Source: CAD feature listing. Evaluate the final solid. Frame: model axes, mm. A direction names the side the tool comes from. Give positions to 0.01 mm unless a question says otherwise; leave off trailing zeros. Order: outer loops, then holes, each group sorted by start corner. A loop starts at its lowest first (then second) coordinate and runs counter-clockwise, first axis right, second up.
from build123d import *

# Parameters (mm, degrees)
SKETCH1_R           = 10
SKETCH1_R_2         = 5.5
BOSS_EXTRUDE1_DEPTH = 2
SKETCH3_R           = 3
BOSS_EXTRUDE2_DEPTH = 12
SKETCH4_R           = 10
SKETCH4_R_2         = 3
BOSS_EXTRUDE3_DEPTH = 2
CHAMFER2_SIZE       = 1
CHAMFER4_SIZE       = 0.5
CUT_EXTRUDE1_REACH  = 6
SKETCH5_R           = 0.75
SKETCH6_R           = 6.25
SKETCH6_R_2         = 5.5
BOSS_EXTRUDE4_DEPTH = 26
CUT_EXTRUDE2_REACH  = 32
SKETCH7_R           = 0.75
SKETCH9_R           = 17.358770913
CUT_EXTRUDE3_DEPTH  = 28


with BuildPart() as part:
    # Sketch1 → Boss-Extrude1 (new body)
    with BuildSketch(Plane.XY):
        Circle(SKETCH1_R)
        Circle(SKETCH1_R_2, mode=Mode.SUBTRACT)
    extrude(amount=BOSS_EXTRUDE1_DEPTH)



with BuildPart() as body_2:
    # Sketch3 → Boss-Extrude2 (new body)
    with BuildSketch(Plane(origin=(0, 0, 0), x_dir=(-1, 0, 0), z_dir=(0, 0, -1))):
        Circle(SKETCH3_R)
    extrude(amount=BOSS_EXTRUDE2_DEPTH)


with BuildPart() as part_1:
    add(part.part)

    add(body_2.part)  # Boss-Extrude3 merges body 2
    # Sketch4 → Boss-Extrude3 (add)
    with BuildSketch(Plane(origin=(0, 0, 0), x_dir=(-1, 0, 0), z_dir=(0, 0, -1))):
        Circle(SKETCH4_R)
        Circle(SKETCH4_R_2, mode=Mode.SUBTRACT)
    extrude(amount=BOSS_EXTRUDE3_DEPTH)

    # Chamfer2
    chamfer2_edges = [part_1.edges().sort_by_distance(p)[0] for p in [
        (3, 0, -2),
    ]]
    chamfer(chamfer2_edges, length=CHAMFER2_SIZE)

    # Chamfer4
    chamfer4_edges = [part_1.edges().sort_by_distance(p)[0] for p in [
        (3, 0, -12),
    ]]
    chamfer(chamfer4_edges, length=CHAMFER4_SIZE)

    # Sketch5 → Cut-Extrude1 (cut, up to next)
    with BuildSketch(Plane(origin=(0, 0, -2), x_dir=(-1, 0, 0), z_dir=(0, 0, -1)), mode=Mode.PRIVATE) as cut_extrude1_sk1:
        with Locations((-8.5, 0)):
            Circle(SKETCH5_R)
    cut_extrude1_tool1 = extrude(cut_extrude1_sk1.sketch, amount=-CUT_EXTRUDE1_REACH, mode=Mode.PRIVATE) & part_1.part
    add(cut_extrude1_tool1.solids().sort_by_distance((8.5, 0, -2))[0], mode=Mode.SUBTRACT)
    # Sketch5 → Cut-Extrude1 (cut, up to next)
    with BuildSketch(Plane(origin=(0, 0, -2), x_dir=(-1, 0, 0), z_dir=(0, 0, -1)), mode=Mode.PRIVATE) as cut_extrude1_sk2:
        with Locations((8.5, 0)):
            Circle(SKETCH5_R)
    cut_extrude1_tool2 = extrude(cut_extrude1_sk2.sketch, amount=-CUT_EXTRUDE1_REACH, mode=Mode.PRIVATE) & part_1.part
    add(cut_extrude1_tool2.solids().sort_by_distance((-8.5, 0, -2))[0], mode=Mode.SUBTRACT)

    # Sketch6 → Boss-Extrude4 (add)
    with BuildSketch(Plane.XY.offset(2)):
        Circle(SKETCH6_R)
        Circle(SKETCH6_R_2, mode=Mode.SUBTRACT)
    extrude(amount=BOSS_EXTRUDE4_DEPTH)

    # Sketch7 → Cut-Extrude2 (cut, up to next)
    with BuildSketch(Plane(origin=(0, 0, -2), x_dir=(-1, 0, 0), z_dir=(0, 0, -1)), mode=Mode.PRIVATE) as cut_extrude2_sk1:
        with Locations((0, 7.5)):
            Circle(SKETCH7_R)
    cut_extrude2_tool1 = extrude(cut_extrude2_sk1.sketch, amount=-CUT_EXTRUDE2_REACH, mode=Mode.PRIVATE) & part_1.part
    add(cut_extrude2_tool1.solids().sort_by_distance((0, 7.5, -2))[0], mode=Mode.SUBTRACT)
    # Sketch7 → Cut-Extrude2 (cut, up to next)
    with BuildSketch(Plane(origin=(0, 0, -2), x_dir=(-1, 0, 0), z_dir=(0, 0, -1)), mode=Mode.PRIVATE) as cut_extrude2_sk2:
        with Locations((6.495190528, -3.75)):
            Circle(SKETCH7_R)
    cut_extrude2_tool2 = extrude(cut_extrude2_sk2.sketch, amount=-CUT_EXTRUDE2_REACH, mode=Mode.PRIVATE) & part_1.part
    add(cut_extrude2_tool2.solids().sort_by_distance((-6.495191, -3.75, -2))[0], mode=Mode.SUBTRACT)
    # Sketch7 → Cut-Extrude2 (cut, up to next)
    with BuildSketch(Plane(origin=(0, 0, -2), x_dir=(-1, 0, 0), z_dir=(0, 0, -1)), mode=Mode.PRIVATE) as cut_extrude2_sk3:
        with Locations((-6.495190528, -3.75)):
            Circle(SKETCH7_R)
    cut_extrude2_tool3 = extrude(cut_extrude2_sk3.sketch, amount=-CUT_EXTRUDE2_REACH, mode=Mode.PRIVATE) & part_1.part
    add(cut_extrude2_tool3.solids().sort_by_distance((6.495191, -3.75, -2))[0], mode=Mode.SUBTRACT)

    # Sketch9 → Cut-Extrude3 (cut)
    with BuildSketch(Plane.XY.offset(28)):
        Circle(SKETCH9_R)
    extrude(amount=-CUT_EXTRUDE3_DEPTH, mode=Mode.SUBTRACT)


solid = part_1.part
(1) Draft query along X for faces 3 (the cylindrical face through (2.17, -9.76, -0.99)), 4 (the cylindrical face through (-6.841, -4.415, -1.014)), 5 (the flat face through (0, 0, 0)). Return one class per face: +X half, -X half, draft (parallel to the pull), parting line (faces both ways), or undercut.
(2) Section C-C, the plane y = 7.5. Return loops of the section in (x, z), plus the area to 3 significant figures.
(3) Access query for faces 1 (the cylindrical face through (3, 0, -7)), 2 (the cylindrical face through (9.25, 0.03, -1.01)). Directions: +Z, -Z, +X, -X, +Y, -Y. A direction counts if a zero-diameter tool reaches every point of the face in a straight line with its end or side. Return the directions, or none.
(4) Section D-D, the plane z = -7.25. Return loops of the section in (x, y), plus the area to 3 significant figures.
(5) Pin query (flat end, axial travel): pin 1 Ø1.4 at (x, y) = (6.5, -3.75) entering from -Z; pin 2 Ø2.5 at (x, y) = (-6.5, -3.75) entering from -Z; pin 3 Ø1.5 at (x, y) = (2, 3) entering from -Z; pin 4 Ø2 at (x, z) = (-1.5, -2.5) entering from -Y. Return the tip coordinate at first contact, or that it passes through.
(6) Section A-A, the plane x = 0. Return loops of the section in (y, z), plus the area to 4 significant figures.
(7) Line query: line 1 along Z through (x, y) = (-5.5, -4.75); line 2 along Z through (x, y) = (-1, 3); line 3 along Y through (x, z) = (1.25, -5). Output: solid intervals per line, ascending.
(8) Section B-B, the plane y = 0. Return loops of the section in (x, z).
Checks:
1. face 3: parting line
1. face 4: undercut
1. face 5: draft
2. outline: (-6.61, -2) - (-0.75, -2) - (-0.75, 0) - (-6.61, 0) - close; (0.75, -2) - (6.61, -2) - (6.61, 0) - (0.75, 0) - close
2. area: 23.5 mm2
3. face 1: -Z
3. face 2: +Z, -Z
4. outline: circle Ø6 at (0, 0)
4. area: 28.3 mm2
5. pin 1: passes through
5. pin 2: stops at z = -2
5. pin 3: stops at z = -11.64
5. pin 4: stops at y = -9.98
6. outline: (-10, -2) - (-4, -2) - (-3, -3) - (-3, -11.5) - (-2.5, -12) - (2.5, -12) - (3, -11.5) - (3, -3) - (4, -2) - (6.75, -2) - (6.75, 0) - (-10, 0) - close; (8.25, -2) - (10, -2) - (10, 0) - (8.25, 0) - close
6. area: 97.75 mm2
7. line 1: z = -2 to 0
7. line 2: z = -2.84 to 0
7. line 3: y = -2.73 to 2.73
8. outline: (-10, -2) - (-9.25, -2) - (-9.25, 0) - (-10, 0) - close; (-7.75, -2) - (-4, -2) - (-3, -3) - (-3, -11.5) - (-2.5, -12) - (2.5, -12) - (3, -11.5) - (3, -3) - (4, -2) - (7.75, -2) - (7.75, 0) - (-7.75, 0) - close; (9.25, -2) - (10, -2) - (10, 0) - (9.25, 0) - close
